Autodesk Inventor part; units mm, degrees
ref_plane "Work Plane1" through (70, -19.23, 0) normal (0, -1, 0) x (1, 0, 0)
ref_plane "YZ Plane" through (0, 0, 0) normal (1, 0, 0) x (0, 1, 0)
ref_plane "XZ Plane" through (0, 0, 0) normal (0, 1, 0) x (-1, 0, 0)
sketch "Sketch1" plane through (0, 0, 0) normal (0, 0, 1) x (1, 0, 0)
  line L0 (-70, -20.5) -> (70, -20.5)
  line L1 (70, -20.5) -> (70, 20.5)
  line L2 (70, 20.5) -> (-70, 20.5)
  line L3 (-70, 20.5) -> (-70, -20.5)
  line L4 (-70, -20.5) -> (70, 20.5) construction
  line L5 (70, -20.5) -> (-70, 20.5) construction
  point P0 (0, 0)
  dimension "d0" = 140
  dimension "d1" = 41
extrude "Extrusion1" add sketch "Sketch1" along normal blind 290
sketch "Sketch2" plane through (-70, 20.5, 0) normal (0, 1, 0) x (1, 0, 0)
  line L0 (140, -290) -> (0, -290)
  line L1 (140, 0) -> (0, 0)
  arc A0 (11.25, -286) -> (6.75, -286) centre (9, -286) ccw
  arc A1 (133.25, -286) -> (128.75, -286) centre (131, -286) ccw
  arc A2 (128.75, -4) -> (133.25, -4) centre (131, -4) ccw
  arc A3 (6.75, -4) -> (11.25, -4) centre (9, -4) ccw
  line L2 (9, -286) -> (9, -4) construction
  line L3 (9, -4) -> (131, -4) construction
  line L4 (131, -4) -> (131, -286) construction
  line L5 (9, -286) -> (9, -290) construction
  line L6 (9, -4) -> (9, 0) construction
  line L7 (9, -4) -> (0, 0) construction
  line L8 (131, -4) -> (140, 0) construction
  line L9 (128.75, -286) -> (128.75, -290)
  line L10 (133.25, -286) -> (133.25, -290)
  line L11 (6.75, -286) -> (6.75, -290)
  line L12 (11.25, -286) -> (11.25, -290)
  line L13 (11.25, -4) -> (11.25, 0)
  line L14 (6.75, -4) -> (6.75, 0)
  line L15 (133.25, -4) -> (133.25, 0)
  line L16 (128.75, -4) -> (128.75, 0)
  point P0 (70, 0)
  dimension "d4" = 2.25
  dimension "d5" = 282
  dimension "d6" = 122
extrude "Extrusion2" cut sketch "Sketch2" against normal up to surface (41 mm away)
ref_plane "Work Plane1" through (70, -19.23, 0) normal (0, -1, 0) x (1, 0, 0)
sketch "Sketch3" plane through (-70, 20.5, 290) normal (0, 1, 0) x (1, 0, 0)
  line L0 (0, 290) -> (0, 0)
  line L1 (140, 290) -> (140, 0)
  line L2 (138.73, 0) -> (138.73, 25.4)
  line L3 (138.73, 25.4) -> (1.27, 25.4)
  line L4 (1.27, 25.4) -> (1.27, 0)
  line L5 (1.27, 0) -> (138.73, 0)
  line L6 (1.27, 0) -> (0, 0) construction
  line L7 (140, 0) -> (138.73, 0) construction
  line L8 (1.27, 264.6) -> (138.73, 264.6)
  line L9 (138.73, 264.6) -> (138.73, 290)
  line L10 (138.73, 290) -> (1.27, 290)
  line L11 (1.27, 290) -> (1.27, 264.6)
  line L12 (1.27, 290) -> (0, 290) construction
  point P0 (70, 290)
  dimension "d9" = 1.27
  dimension "d10" = 25.4
extrude "Extrusion3" cut sketch "Sketch3" against normal up to surface (39.73 mm away)
properties part number "UHP-1500-230"
Geometry: final body of the model. Coordinates: model frame, mm. A direction names the side the tool comes from. Round coordinates to 2 decimals unless told otherwise and drop trailing zeros. Order: outer loops, then holes, each group sorted by start corner. A loop starts at its lowest first (then second) coordinate and runs counter-clockwise, first axis right, second up. Notation, with made-up numbers: M 69.5,11.5 L 95.5,11.5 A11 ccw 95.5,30.5 Z; hole C -28.5,-38.75 d2. An arc over 180 degrees is marked long. One line per item, written item: value.
(1) Pull-direction query (X, two-part tool) for faces 4 (the flat face through (69, -3, 290)), 5 (the flat face through (-1, -19.23, 277)), 6 (the flat face through (70, 0, 143)); classes: pulls with the +X half, pulls with the -X half, needs draft (parallel to the pull), parting line crosses it, or undercut.
Result sheet:
face 4: needs draft
face 5: undercut
face 6: pulls with the +X half
(2) Line query: probe 1 along Y at (x, z) = (-8, 271); probe 2 along Z at (x, y) = (8, 4); probe 3 along X at (y, z) = (0.5, 269). Output: solid intervals per line, ascending. Write a range as [from, to].
Result sheet:
probe 1: [-20.5, -19.23]
probe 2: [25.4, 264.6]
probe 3: [-70, -68.73], [68.73, 70]
(3) Cut plane A-A (y = -9.5). Return the cut outline in (x, z).
Result sheet:
outline: M -70,0 L -68.73,0 L -68.73,25.4 L 68.73,25.4 L 68.73,0 L 70,0 L 70,290 L 68.73,290 L 68.73,264.6 L -68.73,264.6 L -68.73,290 L -70,290 Z
(4) Reachability of faces 1 (the flat face through (-68.73, 1, 277)), 2 (the flat face through (-1, 1, 25.4)), 3 (the flat face through (-69, -3, 0)) from +Z, -Z, +X, -X, +Y, -Y: full face, straight path, thin tool, end or side. Return the list, or none.
Result sheet:
face 1: +Z, +Y
face 2: -Z, +Y
face 3: -Z, +X, -X, +Y, -Y
(5) Pin query (flat end, axial travel): P1, Ø3, axis at x = -16, y = 16.5, coming from the +Z side; P2, Ø12.5, axis at x = -7, z = 283, coming from the +Y side; P3, Ø1.5, axis at x = -6, y = -11, coming from the -Z side. Return the tip coordinate at first contact, or that it passes through.
Result sheet:
P1: z = 264.6
P2: y = -19.23
P3: z = 25.4
(6) Cut plane B-B (x = -13). Return the cut outline in (y, z), and give its area (3 significant figures).
Result sheet:
outline: M -20.5,0 L -19.23,0 L -19.23,25.4 L 20.5,25.4 L 20.5,264.6 L -19.23,264.6 L -19.23,290 L -20.5,290 Z
area: 9,870 mm2
(7) Cut plane C-C (z = 272.5). Return the cut outline in (x, y), and give its area (3 significant figures).
Result sheet:
outline: M -70,-20.5 L 70,-20.5 L 70,20.5 L 68.73,20.5 L 68.73,-19.23 L -68.73,-19.23 L -68.73,20.5 L -70,20.5 Z
area: 279 mm2
